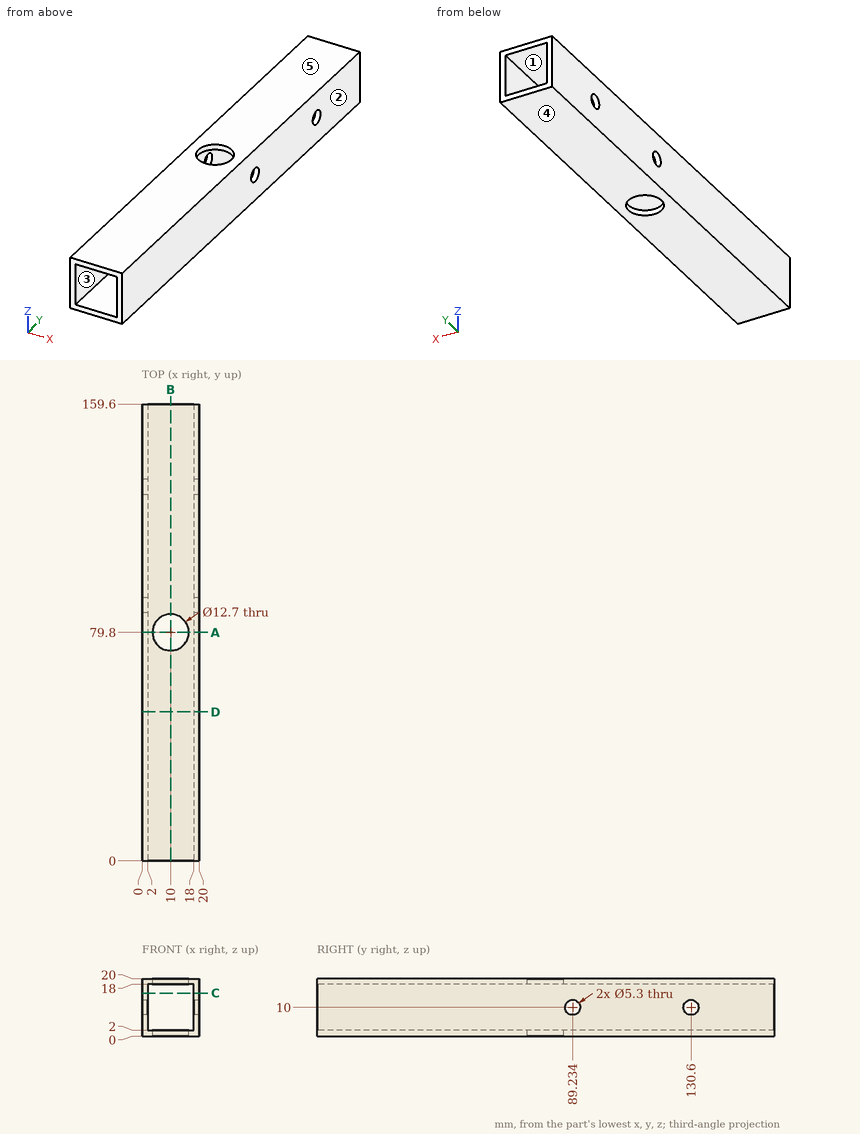
Job drawing, mm, ordinate dimensions from the low corner. One solid piece. A direction names the side the tool comes from. Give positions to 0.01 mm unless a question says otherwise; leave off trailing zeros. Loops run counter-clockwise (first coordinate to the right, second up) from the corner with the lowest first, then second, coordinate; pieces in that order, holes last. Notation, with made-up numbers: M -7.75,70 L 22.25,70 A27 cw 22.25,97 Z; hole C 56.25,8.25 d2. An arc over 180 degrees is marked long. Answer in a Markdown table with one row per item. Add a question column.
Item 1: Mould opens along Z. For the marked faces 3, 4 and 5 say: +Z half, -Z half, draft (parallel to the pull), parting line (faces both ways), or undercut.
Item 2: Probe probe 1 along Y at (x, z) = (0.9, 10); probe 2 along Z at (x, y) = (19.3, 130.6); probe 3 along Z at (x, y) = (15.75, 40). List the from-to ranges inside material, lowest first.
Item 3: Band-saw the part on A-A on y = 79.8. Give the cut face in (x, z).
Item 4: Tool access for the marked faces 1 and 2: list every direction of +Z, -Z, +X, -X, +Y, -Y with a clear straight run to the whole face (end or side of a thin tool).
Item 5: Band-saw the part on D-D on y = 52. Give the cut face in (x, z), then the cut area to 3 significant figures.
Item 6: Band-saw the part on B-B on x = 10. Give the cut face in (y, z).
Item 7: Band-saw the part on C-C on z = 15. Give the cut face in (x, y).
Item 8: Drop a flat-ended pin along its axis: P1, Ø1, axis at x = 16.5, z = 13, coming from the +Y side. Give the stop position or say it passes through.
Reply:
| question | item | result |
|---|---|---|
| 1 | face 3 | undercut |
| 1 | face 4 | -Z half |
| 1 | face 5 | +Z half |
| 2 | probe 1 | y = 0 to 86.58, 91.88 to 127.95, 133.25 to 159.6 |
| 2 | probe 2 | z = 0 to 7.35, 12.65 to 20 |
| 2 | probe 3 | z = 0 to 2, 18 to 20 |
| 3 | outline | M 0,0 L 3.65,0 L 3.65,2 L 2,2 L 2,18 L 3.65,18 L 3.65,20 L 0,20 Z; M 16.35,0 L 20,0 L 20,20 L 16.35,20 L 16.35,18 L 18,18 L 18,2 L 16.35,2 Z |
| 4 | face 1 | +Y, -Y |
| 4 | face 2 | +Z, -Z, +X, +Y, -Y |
| 5 | outline | M 0,0 L 20,0 L 20,20 L 0,20 Z; hole M 2,2 L 18,2 L 18,18 L 2,18 Z |
| 5 | area | 144 mm^2 |
| 6 | outline | M 0,0 L 73.45,0 L 73.45,2 L 0,2 Z; M 0,18 L 73.45,18 L 73.45,20 L 0,20 Z; M 86.15,0 L 159.6,0 L 159.6,2 L 86.15,2 Z; M 86.15,18 L 159.6,18 L 159.6,20 L 86.15,20 Z |
| 7 | outline | M 0,0 L 2,0 L 2,159.6 L 0,159.6 Z; M 18,0 L 20,0 L 20,159.6 L 18,159.6 Z |
| 8 | P1 | passes through |
